Autodesk Inventor part; units mm, degrees
ref_plane "YZ Plane" through (0, 0, 0) normal (1, 0, 0) x (0, 1, 0)
ref_plane "XZ Plane" through (0, 0, 0) normal (0, 1, 0) x (-1, 0, 0)
ref_plane "XY Plane" through (0, 0, 0) normal (0, 0, 1) x (1, 0, 0)
sketch "Sketch1" plane through (0, 0, 0) normal (0, 1, 0) x (-1, 0, 0)
  line L0 (0, 0) -> (40, 0)
  line L1 (40, 0) -> (40, -50)
  line L2 (40, -50) -> (0, -50)
  line L3 (0, -50) -> (0, 0)
  line L4 (40, 0) -> (0, 0)
  line L5 (0, 0) -> (0, -18)
  line L6 (5, -18) -> (35, -18)
  line L7 (40, -18) -> (40, 0)
  line L8 (35, -18) -> (5, -18)
  line L9 (0, -18) -> (0, -37)
  line L10 (5, -37) -> (35, -37)
  line L11 (40, -37) -> (40, -18)
  circle A0 centre (20, -7) radius 1.7
  circle A1 centre (20, -43) radius 1.7
  line L12 (20, -18) -> (35, -18)
  line L13 (35, -18) -> (35, -37)
  line L14 (35, -37) -> (20, -37)
  line L15 (20, -37) -> (5, -37)
  line L16 (5, -37) -> (5, -18)
  line L17 (5, -18) -> (20, -18)
  line L18 (35, -21) -> (5, -21)
  line L19 (5, -21) -> (5, -34)
  line L20 (5, -34) -> (35, -34)
  line L21 (35, -34) -> (35, -21)
  dimension "d0" = 40
  dimension "d1" = 50
  dimension "d2" = 3.4
  dimension "d3" = 3.4
  dimension "d6" = 19
extrude "Extrusion1" add sketch "Sketch1" along normal blind 5 contours L0 L1 L2 L3 | L6 L13 L18 L16 | L20 L13 L10 L16
properties part number "_3DPrint"
CAD build for the part. Positions are in the model's coordinates, mm. A direction names the side the tool comes from. Coordinates: 2 decimals unless noted, no trailing zeros. Order: outer loops, then holes, each group sorted by start corner. A loop starts at its lowest first (then second) coordinate and runs counter-clockwise, first axis right, second up. Notation, with made-up numbers: (84, 9.25) -> (115, 9.25) arc R29 ccw to (115, 46.25) -> close; hole circle Ø7 at (44.25, 70.5). An arc over 180 degrees is marked (long way). Use one line per item in the form item = value. Start each with the question number.
1) Band-saw the part on D-D on x = -20. Give the cut face in (y, z).
2) Band-saw the part on B-B on z = -26. Give the cut face in (x, y).
3) Tool access for faces 4 (the flat face through (-20, 2, -21)), 5 (the flat face through (0, 2, -25)): list every direction of +Z, -Z, +X, -X, +Y, -Y with a clear straight run to the whole face (end or side of a thin tool).
4) Band-saw the part on C-C on y = 1.2. Give the cut face in (x, z).
5) Pull direction Z, two halves, no side cores. Call faces 1 (the flat face through (-40, 2, -25)), 2 (the flat face through (-20, 2, 0)), 3 (the cylindrical face through (-20.8, 2.5, -41.5)): +Z half, -Z half, draft (parallel to the pull), parting line (faces both ways), or undercut.
6) Drill centre lines: L1, parallel to Z at x = -20, y = 1.55; L2, parallel to Z at x = -32, y = 3.25; L3, parallel to X at y = 2.85, z = -27.5. Where is each one in solid material? Low to high. Write a range as [from, to].
7) Band-saw the part on A-A on x = -6. Give the cut face in (y, z), then the cut area to 3 significant figures.
Entries:
q1.outline = (0, -50) -> (5, -50) -> (5, -44.7) -> (0, -44.7) -> close; (0, -41.3) -> (5, -41.3) -> (5, -34) -> (0, -34) -> close; (0, -21) -> (5, -21) -> (5, -8.7) -> (0, -8.7) -> close; (0, -5.3) -> (5, -5.3) -> (5, 0) -> (0, 0) -> close
q2.outline = (-40, 0) -> (-35, 0) -> (-35, 5) -> (-40, 5) -> close; (-5, 0) -> (0, 0) -> (0, 5) -> (-5, 5) -> close
q3.face_4 = +Y, -Y
q3.face_5 = +Z, -Z, +X, +Y, -Y
q4.outline = (-40, -50) -> (0, -50) -> (0, 0) -> (-40, 0) -> close; hole (-35, -34) -> (-5, -34) -> (-5, -21) -> (-35, -21) -> close; hole circle Ø3.4 at (-20, -43); hole circle Ø3.4 at (-20, -7)
q5.face_1 = draft
q5.face_2 = +Z half
q5.face_3 = undercut
q6.L1 = [-50, -44.7], [-41.3, -34], [-21, -8.7], [-5.3, 0]
q6.L2 = [-50, -34], [-21, 0]
q6.L3 = [-40, -35], [-5, 0]
q7.outline = (0, -50) -> (5, -50) -> (5, -34) -> (0, -34) -> close; (0, -21) -> (5, -21) -> (5, 0) -> (0, 0) -> close
q7.area = 185 mm2
